Verification items for the finished model (mm, model axes). A direction names the side the tool comes from. Round coordinates to 2 decimals unless told otherwise and drop trailing zeros. Order: outer loops, then holes, each group sorted by start corner. A loop starts at its lowest first (then second) coordinate and runs counter-clockwise, first axis right, second up. Notation, with made-up numbers: M -7,0.25 L 16,0.25 A18 cw 16,25.25 Z; hole C -20.5,-39.5 d10. An arc over 180 degrees is marked long. Write item = value, one per line. Start each with the question number.
Autodesk Inventor part; units mm, degrees
ref_plane "YZ Plane" through (0, 0, 0) normal (1, 0, 0) x (0, 1, 0)
ref_plane "XZ Plane" through (0, 0, 0) normal (0, 1, 0) x (-1, 0, 0)
ref_plane "XY Plane" through (0, 0, 0) normal (0, 0, 1) x (1, 0, 0)
sketch "Sketch1" plane through (0, 0, 0) normal (0, 1, 0) x (-1, 0, 0)
  line L0 (0, 0) -> (76.2, 0)
  line L1 (76.2, 0) -> (76.2, -114.3)
  line L2 (76.2, -114.3) -> (0, -114.3)
  line L3 (0, -114.3) -> (0, 0)
  dimension "d0" = 76.2
  dimension "d1" = 114.3
extrude "Extrusion1" add sketch "Sketch1" along normal blind 3.175
sketch "Sketch2" plane through (0, 3.175, 0) normal (0, 1, 0) x (1, 0, 0)
  line L0 (0, 12.7) -> (3.175, 12.7)
  line L1 (3.175, 12.7) -> (3.175, 31.75)
  line L2 (3.175, 31.75) -> (0, 31.75)
  line L3 (0, 31.75) -> (0, 12.7)
  line L4 (0, 0) -> (0, 114.3)
  line L5 (0, 82.55) -> (3.175, 82.55)
  line L6 (3.175, 82.55) -> (3.175, 101.6)
  line L7 (3.175, 101.6) -> (0, 101.6)
  line L8 (0, 101.6) -> (0, 82.55)
  line L9 (-76.2, 0) -> (0, 0)
  line L10 (0, 114.3) -> (-76.2, 114.3)
  line L11 (-38.1, 0) -> (-38.1, 114.3)
  line L12 (-76.2, 12.7) -> (-79.375, 12.7)
  line L13 (-79.375, 12.7) -> (-79.375, 31.75)
  line L14 (-79.375, 31.75) -> (-76.2, 31.75)
  line L15 (-76.2, 31.75) -> (-76.2, 12.7)
  line L16 (-76.2, 0) -> (-76.2, 114.3)
  line L17 (-76.2, 82.55) -> (-79.375, 82.55)
  line L18 (-79.375, 82.55) -> (-79.375, 101.6)
  line L19 (-79.375, 101.6) -> (-76.2, 101.6)
  line L20 (-76.2, 101.6) -> (-76.2, 82.55)
  dimension "d4" = 19.05
  dimension "d5" = 19.05
  dimension "d6" = 12.7
  dimension "d7" = 12.7
  dimension "d8" = 3.175
  dimension "d9" = 3.175
  dimension "d10" = 0
extrude "Extrusion2" add sketch "Sketch2" against normal blind 3.175 contours L3 L2 L1 L0 | L4 L7 L6 L5 | L12 L13 L14 L15 | L16 L17 L18 L19
sketch "Sketch3" plane through (0, 3.175, 0) normal (0, 1, 0) x (1, 0, 0)
  line L0 (0, 82.55) -> (0, 31.75)
  line L1 (0, 38.1) -> (-31.75, 38.1)
  line L2 (-31.75, 38.1) -> (-31.75, 76.2)
  line L3 (-31.75, 76.2) -> (0, 76.2)
  line L4 (0, 76.2) -> (0, 38.1)
  line L5 (0, 82.55) -> (3.175, 82.55)
  line L6 (3.175, 31.75) -> (0, 31.75)
  line L7 (-76.2, 0) -> (0, 0)
  line L8 (-38.1, 0) -> (-38.1, 114.3) construction
  line L9 (0, 114.3) -> (-76.2, 114.3)
  line L10 (-76.2, 82.55) -> (-76.2, 31.75)
  line L11 (-76.2, 38.1) -> (-44.45, 38.1)
  line L12 (-44.45, 38.1) -> (-44.45, 76.2)
  line L13 (-44.45, 76.2) -> (-76.2, 76.2)
  line L14 (-76.2, 76.2) -> (-76.2, 38.1)
  line L15 (-76.2, 82.55) -> (-79.375, 82.55)
  line L16 (-79.375, 31.75) -> (-76.2, 31.75)
  dimension "d13" = 6.35
  dimension "d14" = 6.35
  dimension "d15" = 31.75
extrude "Extrusion3" cut sketch "Sketch3" against normal blind 3.175
sketch "Sketch4" plane through (0, 3.175, 0) normal (0, 1, 0) x (1, 0, 0)
  circle A0 centre (-22.86, 84.68) radius 2.2225
  circle A1 centre (-22.86, 108.81) radius 2.2225
  circle A2 centre (-53.34, 108.81) radius 2.2225
  line L0 (-31.75, 57.15) -> (-44.45, 57.15) construction
  line L1 (0, 101.6) -> (0, 114.3)
  circle A3 centre (-53.34, 84.68) radius 2.2225
  circle A4 centre (-22.86, 29.62) radius 2.2225
  circle A5 centre (-22.86, 5.49) radius 2.2225
  circle A6 centre (-53.34, 5.49) radius 2.2225
  circle A7 centre (-53.34, 29.62) radius 2.2225
  point P0 (0, 0)
  dimension "d24" = 4.445
  dimension "d25" = 4.445
  dimension "d26" = 4.445
  dimension "d30" = 24.13
  dimension "d33" = 30.48
  dimension "d36" = 30.48
  dimension "d37" = 22.86
  dimension "d38" = 4.445
extrude "Extrusion4" cut sketch "Sketch4" against normal blind 3.175
sketch "Sketch5" plane through (0, 3.175, 0) normal (0, 1, 0) x (1, 0, 0)
  line L0 (-36.5125, 5.08) -> (-39.6875, 5.08)
  line L1 (-39.6875, 5.08) -> (-39.6875, 35.56)
  line L2 (-39.6875, 35.56) -> (-36.5125, 35.56)
  line L3 (-36.5125, 35.56) -> (-36.5125, 5.08)
  line L4 (-36.5125, 78.74) -> (-39.6875, 78.74)
  line L5 (-39.6875, 78.74) -> (-39.6875, 109.22)
  line L6 (-39.6875, 109.22) -> (-36.5125, 109.22)
  line L7 (-36.5125, 109.22) -> (-36.5125, 78.74)
  line L8 (-76.2, 0) -> (0, 0)
  line L9 (0, 114.3) -> (-76.2, 114.3)
  line L10 (0, 101.6) -> (0, 114.3)
  dimension "d39" = 3.175
  dimension "d40" = 5.08
  dimension "d41" = 5.08
  dimension "d42" = 30.48
  dimension "d43" = 30.48
  dimension "d44" = 36.5125
extrude "Extrusion5" cut sketch "Sketch5" against normal blind 3.175
properties part number "base"
1) Cross-section at D-D, the plane x = -68. Enter the section's corners in (y, z) (3 decimals), then the cut area to 3 significant figures.
2) Cross-section at B-B, the plane z = -20. Enter the section's corners in (x, y) (1 decimal).
3) Scan lines: probe 1 along X at (y, z) = (1.2, -108.81); probe 2 along X at (y, z) = (2.1, -84.68) (1 decimal); probe 3 along X at (y, z) = (0.35, -26.5) (1 decimal). Record each from-to range of solid material in increasing order.
4) Gauge pin test, flat ends, axial feed: P1, Ø1, axis at x = -28, z = -100.5, coming from the -Y side; P2, Ø1, axis at y = 2.5, z = -105, coming from the +X side; P3, Ø1, axis at x = 2, y = 2, coming from the +Z side; P4, Ø1.6, axis at x = 1, y = 1.5, coming from the -Z side. Record the tip position at first contact, or that the pin passes through.
5) Cross-section at C-C, the plane z = -84.68. Enter the section's corners in (x, y) (1 decimal).
6) Access from +Z, -Z, +X, -X, +Y, -Y to the whole of each face (thin tool, end or side, straight path). Record for faces 1 (the flat face through (2, 2, -12.7)), 2 (the flat face through (-39.688, 2, -20)), 3 (the flat face through (-78, 2, -101.6)), 4 (the flat face through (2, 2, -101.6)), 5 (the flat face through (2, 2, -82.55)).
7) Cross-section at A-A, the plane x = -22.86. Enter the section's corners in (y, z) (1 decimal), then the cut area to 3 significant figures.
8) Release check for a two-part mould opening along X. For faces 6 (the flat face through (-38, 2, -35.56)), 7 (the flat face through (-76.2, 2, -79)), 8 (the flat face through (-78, 2, -82.55)) record: pulls with the +X half, pulls with the -X half, needs draft (parallel to the pull), parting line crosses it, or undercut.
Geometry results:
q1.outline = M 0,-114.3 L 3.175,-114.3 L 3.175,-76.2 L 0,-76.2 Z; M 0,-38.1 L 3.175,-38.1 L 3.175,0 L 0,0 Z
q1.area = 242 mm^2
q2.outline = M -79.4,0 L -39.7,0 L -39.7,3.2 L -79.4,3.2 Z; M -36.5,0 L 3.2,0 L 3.2,3.2 L -36.5,3.2 Z
q3.probe_1 = -76.2 to -55.56, -51.12 to -39.69, -36.51 to -25.08, -20.64 to 0
q3.probe_2 = -79.4 to -55.6, -51.1 to -39.7, -36.5 to -25.1, -20.6 to 3.2
q3.probe_3 = -79.4 to -39.7, -36.5 to 3.2
q4.P1 = 0
q4.P2 = 0
q4.P3 = -12.7
q4.P4 = -101.6
q5.outline = M -79.4,0 L -55.6,0 L -55.6,3.2 L -79.4,3.2 Z; M -51.1,0 L -39.7,0 L -39.7,3.2 L -51.1,3.2 Z; M -36.5,0 L -25.1,0 L -25.1,3.2 L -36.5,3.2 Z; M -20.6,0 L 3.2,0 L 3.2,3.2 L -20.6,3.2 Z
q6.face_1 = +Z, +X, +Y, -Y
q6.face_2 = +Y, -Y
q6.face_3 = -Z, -X, +Y, -Y
q6.face_4 = -Z, +X, +Y, -Y
q6.face_5 = +X, +Y, -Y
q7.outline = M 0,-114.3 L 3.2,-114.3 L 3.2,-111 L 0,-111 Z; M 0,-106.6 L 3.2,-106.6 L 3.2,-86.9 L 0,-86.9 Z; M 0,-82.5 L 3.2,-82.5 L 3.2,-76.2 L 0,-76.2 Z; M 0,-38.1 L 3.2,-38.1 L 3.2,-31.8 L 0,-31.8 Z; M 0,-27.4 L 3.2,-27.4 L 3.2,-7.7 L 0,-7.7 Z; M 0,-3.3 L 3.2,-3.3 L 3.2,0 L 0,0 Z
q7.area = 185 mm^2
q8.face_6 = undercut
q8.face_7 = pulls with the -X half
q8.face_8 = needs draft
